Check sheet for the modelled part. Datum: model origin and axes. Units: mm. Face numbers are marked on the shaded views. Give positions to 0.01 mm unless a question says otherwise; leave off trailing zeros. Write each loop counter-clockwise with the first axis right and the second up, starting at its lowest first coordinate (ties: lowest second). Pieces come first, ordered by that corner, then holes. Notation, with made-up numbers: (24.5, 75.5) -> (34.5, 75.5) arc R24 ccw to (34.5, 104.5) -> close; hole circle Ø2 at (0.25, 24). An arc over 180 degrees is marked (long way). Return JSON: item names as keys, results as strings.
from build123d import *

# Parameters (mm, degrees)
ESBO_O1_W                = 200
ESBO_O1_H                = 110
RESSALTO_EXTRUS_O1_DEPTH = 15
ESBO_O7_R                = 3
RESSALTO_EXTRUS_O2_DEPTH = 8


with BuildPart() as part:
    # Esboço1 → Ressalto-extrusão1 (new body)
    with BuildSketch(Plane.XY):
        with Locations((100, 55)):
            Rectangle(ESBO_O1_W, ESBO_O1_H)
    extrude(amount=RESSALTO_EXTRUS_O1_DEPTH)

    # Esboço7 → Ressalto-extrusão2 (add)
    with BuildSketch(Plane(origin=(0, 110, 0), x_dir=(1, 0, 0), z_dir=(0, 1, 0))):
        with Locations((175, -7.5)):
            Circle(ESBO_O7_R)
        with Locations((25, -7.5)):
            Circle(ESBO_O7_R)
    extrude(amount=RESSALTO_EXTRUS_O2_DEPTH)


solid = part.part
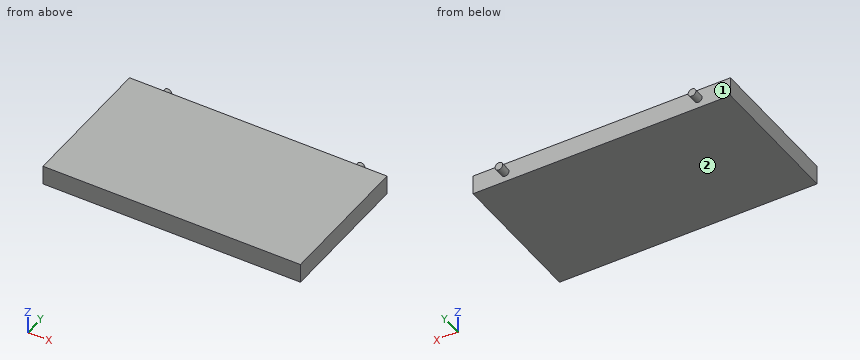
(1) Release check for a two-part mould opening along X. For the marked faces 1 and 2 record: pulls with the +X half, pulls with the -X half, needs draft (parallel to the pull), parting line crosses it, or undercut.
Reply:
{"face 1": "undercut", "face 2": "needs draft"}
(2) Cross-section at B-B on x = 25. Enter the section's corners in (y, z), then the cut area to 3 significant figures.
Reply:
{"outline": "(0, 0) -> (110, 0) -> (110, 4.5) -> (118, 4.5) -> (118, 10.5) -> (110, 10.5) -> (110, 15) -> (0, 15) -> close", "area": "1,700 mm^2"}
(3) Depth check by flat-ended pin: pin 1 Ø2 at (x, z) = (40, 8.5) entering from +Y. Enter the tip coordinate at first touch or a pass-through.
Reply:
{"pin 1": "y = 110"}
(4) Cross-section at A-A on z = 7.5. Enter the section's corners in (x, y), then the cut area to 3 significant figures.
Reply:
{"outline": "(0, 0) -> (200, 0) -> (200, 110) -> (178, 110) -> (178, 118) -> (172, 118) -> (172, 110) -> (28, 110) -> (28, 118) -> (22, 118) -> (22, 110) -> (0, 110) -> close", "area": "22,100 mm^2"}
(5) Thickness scan on L1, parallel to Y at x = 64.5, z = 5. Record the ranges inside material, lowest first.
Reply:
{"L1": "0 to 110"}
(6) Cross-section at C-C on x = 142. Enter the section's corners in (y, z).
Reply:
{"outline": "(0, 0) -> (110, 0) -> (110, 15) -> (0, 15) -> close"}
